Can you work these out from the model? Positions are in its coordinate system, mm. A direction names the side the tool comes from. Give positions to 0.01 mm unless a question says otherwise; leave off trailing zeros. Write each loop counter-clockwise with the first axis right and the second up, starting at its lowest first coordinate (ties: lowest second). Pieces come first, ordered by that corner, then holes. Notation, with made-up numbers: M 86.25,19 L 110.25,19 A32 ccw 110.25,58 Z; hole C 88,56.5 d2. An arc over 180 degrees is marked long. Write each question's results on one line, items separated by ' | '.
from build123d import *

# Parameters (mm, degrees)
F1_DEPTH = 25.4
F2_DEPTH = 25.4
F3_R     = 6.35
F4_DEPTH = 25.4
F5_R     = 5.08


with BuildPart() as f1:
    # F0 (on Front) → F1 (new body)
    with BuildSketch(Plane.XZ):
        with BuildLine():
            ThreePointArc((0, 9.525), (-9.525, 0), (0, -9.525))
            ThreePointArc((0, -9.525), (6.735192, -6.735192), (9.525, 0))
            ThreePointArc((9.525, 0), (6.735192, 6.735192), (0, 9.525))
        make_face()
    extrude(amount=-F1_DEPTH)

    # F0 (on Front) → F2 (join)
    with BuildSketch(Plane.XZ):
        with BuildLine():
            Line((-12.7, 9.525), (-12.7, -9.525))
            Line((-12.7, -9.525), (0, -9.525))
            ThreePointArc((0, -9.525), (-9.525, 0), (0, 9.525))
            Line((0, 9.525), (-12.7, 9.525))
        make_face()
        with BuildLine():
            ThreePointArc((9.525, 0), (6.735192, -6.735192), (0, -9.525))
            Line((0, -9.525), (12.7, -9.525))
            Line((12.7, -9.525), (12.7, 9.525))
            Line((12.7, 9.525), (0, 9.525))
            ThreePointArc((0, 9.525), (6.735192, 6.735192), (9.525, 0))
        make_face()
        with BuildLine():
            ThreePointArc((0, 9.525), (-9.525, 0), (0, -9.525))
            ThreePointArc((0, -9.525), (6.735192, -6.735192), (9.525, 0))
            ThreePointArc((9.525, 0), (6.735192, 6.735192), (0, 9.525))
        make_face()
    extrude(amount=F2_DEPTH)

    # F3 (on face) → F4 (cut)
    with BuildSketch(Plane.XY.offset(9.525)):
        with Locations((0, -17.237177)):
            Circle(F3_R)
    extrude(amount=-F4_DEPTH, mode=Mode.SUBTRACT)

    # F5
    f5_edges = [f1.edges().sort_by_distance(p)[0] for p in [
        (-12.7, -25.4, 0),
        (12.7, -25.4, 0),
    ]]
    fillet(f5_edges, radius=F5_R)


solid = f1.part
Item 1: I want a section at C-C, the plane x = -2.5. Please give me the cut outline in (y, z) (3 decimals), and give its area (3 significant figures).
Geometry says:
outline: M -25.4,-9.525 L -23.074,-9.525 L -23.074,9.525 L -25.4,9.525 Z; M -11.4,-9.525 L 0,-9.525 L 0,-9.191 L 25.4,-9.191 L 25.4,9.191 L 0,9.191 L 0,9.525 L -11.4,9.525 Z | area: 728 mm2
Item 2: I want a section at A-A, the plane y = -19.5. Please give me the cut outline in (x, z) (3 decimals).
Geometry says:
outline: M -12.7,-9.525 L -5.933,-9.525 L -5.933,9.525 L -12.7,9.525 Z; M 5.933,-9.525 L 12.7,-9.525 L 12.7,9.525 L 5.933,9.525 Z
Item 3: I want a section at B-B, the plane z = -4.25. Please give me the cut outline in (x, y).
Geometry says:
outline: M -12.7,-20.32 A5.08 ccw -7.62,-25.4 L 7.62,-25.4 A5.08 ccw 12.7,-20.32 L 12.7,0 L 8.52,0 L 8.52,25.4 L -8.52,25.4 L -8.52,0 L -12.7,0 Z; hole C 0,-17.24 d12.7
Item 4: I want a section at D-D, the plane z = 1.25. Please give me the cut outline in (x, y), and give its area (3 significant figures).
Geometry says:
outline: M -12.7,-20.32 A5.08 ccw -7.62,-25.4 L 7.62,-25.4 A5.08 ccw 12.7,-20.32 L 12.7,0 L 9.44,0 L 9.44,25.4 L -9.44,25.4 L -9.44,0 L -12.7,0 Z; hole C 0,-17.24 d12.7 | area: 987 mm2
Item 5: For faces 1 (the face through (-12.7, -10, 0)), 2 (the face through (-11, 0, 0)), 3 (the face through (10, 0, 0)), which set-ups out of +Z, -Z, +X, -X, +Y, -Y let a thin tool reach every point of the face, with its end or its side?
Geometry says:
face 1: +Z, -Z, -X, +Y, -Y | face 2: -X, +Y | face 3: +X, +Y
Item 6: Thinking about a two-plate mould opening in X: for faces 4 (the face through (0, -10, 9.525)), 5 (the face through (11.172, -23.951, 0.133)), 6 (the face through (-1.377, -23.436, 0.133)), which applies, +X half, -X half, draft (parallel to the pull), parting line (faces both ways), or undercut?
Geometry says:
face 4: draft | face 5: +X half | face 6: undercut
Item 7: I'm going to push flat-ended pins straight in: pin 1 (1.5 mm diameter, centred on y = 12, z = -6, fed in from -X); pin 2 (1.5 mm diameter, centred on x = 8.5, y = 11, fed in from -Z); pin 3 (6.5 mm diameter, centred on x = -8.5, z = -4.5, fed in from +Y); pin 4 (3 mm diameter, centred on y = 19.5, z = 1, fed in from -X) (3 decimals). Where does each tip first touch, or does it pass through?
Geometry says:
pin 1: stops at x = -7.95 | pin 2: stops at z = -5.54 | pin 3: stops at y = 25.4 | pin 4: stops at x = -9.525
Item 8: If I drill on line 1 (Y direction, x = 0, z = 3); line 2 (X direction, y = 23.5, z = 0.25); line 3 (X direction, y = -15, z = -5.5), over which ranges is the centre line in solid material (lowest first)? Write a range as from..to.
Geometry says:
line 1: y = -25.4..-23.59, -10.89..25.4 | line 2: x = -9.52..9.52 | line 3: x = -12.7..-5.94, 5.94..12.7
